Study the drawing (mm; zero at the part's minimum x, y, z) and answer. A direction names the side the tool comes from. Coordinates: 2 decimals unless noted, no trailing zeros. Loops run counter-clockwise (first coordinate to the right, second up) from the corner with the lowest first, then second, coordinate; pieces in that order, holes last. Notation, with made-up numbers: (51, -19.5) - (101, -19.5) arc R22 cw to (101, 8.5) - close; hole circle Ø4 at (-7.5, 84). An arc over 180 degrees is marked (long way). Use one line per item in the form item = value.
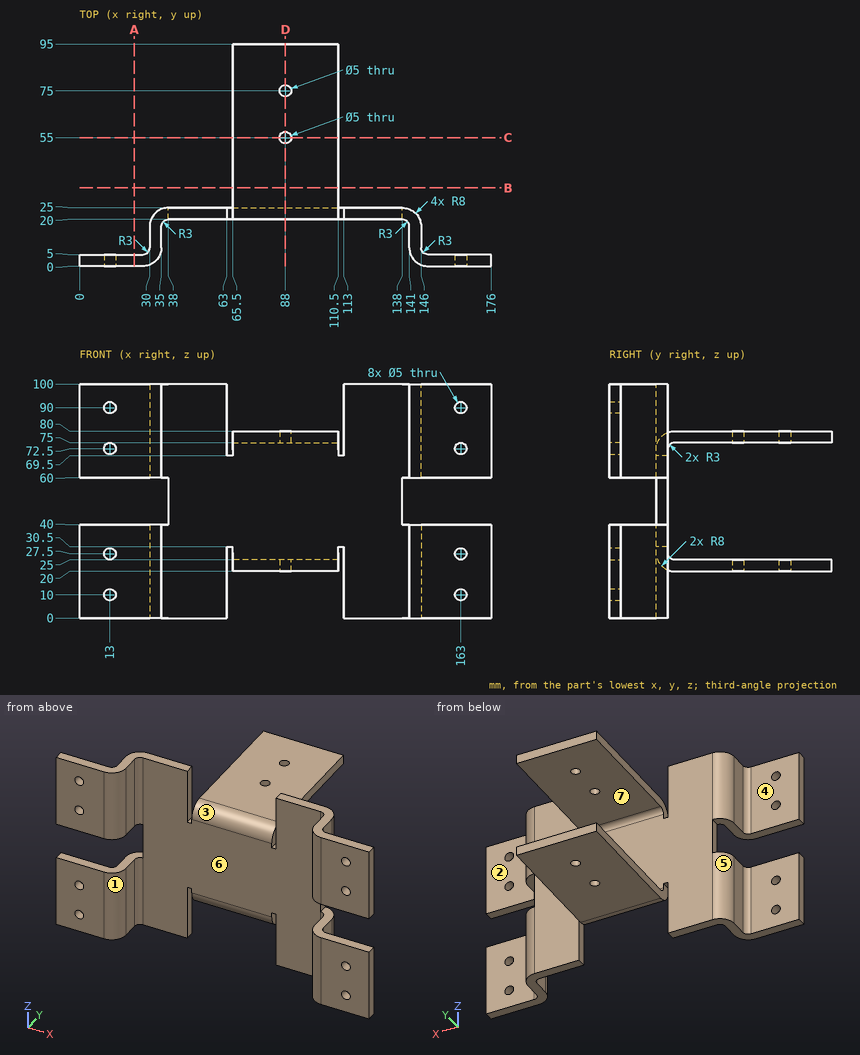
Item 1: Find the intervals of material crossed by L1, parallel to X at y = 3.15, z = 72.5; L2, parallel to Z at x = 108, y = 77.5; L3, parallel to X at y = 3.5, z = 90, in increasing order.
Results below:
L1 = 0 to 10.5, 15.5 to 33.36, 142.64 to 160.5, 165.5 to 176
L2 = 20 to 25, 75 to 80
L3 = 0 to 10.5, 15.5 to 33.61, 142.39 to 160.5, 165.5 to 176
Item 2: The part is cut by section C-C on y = 55. Give the vertices of the cut face in (x, z).
Results below:
outline = (65.5, 20) - (85.5, 20) - (85.5, 25) - (65.5, 25) - close; (65.5, 75) - (85.5, 75) - (85.5, 80) - (65.5, 80) - close; (90.5, 20) - (110.5, 20) - (110.5, 25) - (90.5, 25) - close; (90.5, 75) - (110.5, 75) - (110.5, 80) - (90.5, 80) - close
Item 3: The part is cut by section D-D on x = 88. Give the vertices of the cut face in (y, z), plus the area to 3 significant figures.
Results below:
outline = (20, 28) arc R8 ccw to (28, 20) - (52.5, 20) - (52.5, 25) - (28, 25) arc R3 cw to (25, 28) - (25, 72) arc R3 cw to (28, 75) - (52.5, 75) - (52.5, 80) - (28, 80) arc R8 ccw to (20, 72) - close; (57.5, 20) - (72.5, 20) - (72.5, 25) - (57.5, 25) - close; (57.5, 75) - (72.5, 75) - (72.5, 80) - (57.5, 80) - close; (77.5, 20) - (95, 20) - (95, 25) - (77.5, 25) - close; (77.5, 75) - (95, 75) - (95, 80) - (77.5, 80) - close
area = 876 mm²
Item 4: Each of these flat-tipped pins is pushed along its axis until it touches: P1, Ø4, axis at x = 83, y = 58, coming from the +Z side; P2, Ø5, axis at y = 34.5, z = 74, coming from the -X side; P3, Ø4.5, axis at x = 163, z = 90, coming from the -Y side; P4, Ø1, axis at x = 129, z = 58, coming from the +Y side. Where does it stop, or does it pass through?
Results below:
P1 = 80
P2 = 65.5
P3 = through
P4 = 25
Item 5: The part is cut by section B-B on y = 33.5. Give the vertices of the cut face in (x, z), plus the area to 3 significant figures.
Results below:
outline = (65.5, 20) - (110.5, 20) - (110.5, 25) - (65.5, 25) - close; (65.5, 75) - (110.5, 75) - (110.5, 80) - (65.5, 80) - close
area = 450 mm²
Item 6: Which of the six approach directions +Z, -Z, +X, -X, +Y, -Y give full straight-line access (tool end or side, diameter ignored) to the marked faces 1, 2, 3 and 4?
Results below:
face_1 = +Z, -Z, -Y
face_2 = +Z, -Z, +X, +Y
face_3 = +Z, -Y
face_4 = +Z, -Z, -X, +Y
Item 7: The part is cut by section A-A on x = 23.5. Give the vertices of the cut face in (y, z), plus the area to 3 significant figures.
Results below:
outline = (0, 0) - (5, 0) - (5, 40) - (0, 40) - close; (0, 60) - (5, 60) - (5, 100) - (0, 100) - close
area = 400 mm²
Item 8: For a pull along X with two mould halves and no side action, classify the marked faces 5, 6 and 7 as +X half, -X half, draft (parallel to the pull), parting line (faces both ways), or undercut.
Results below:
face_5 = -X half
face_6 = undercut
face_7 = draft
